Can you work these out from the drawing? Everything is in mm from the part's minimum corner. A direction names the side the tool comes from. Coordinates: 2 decimals unless noted, no trailing zeros. Write each loop counter-clockwise with the first axis right and the second up, starting at its lowest first coordinate (ties: lowest second). Pieces come first, ordered by that corner, then holes.
(1) Which directions (+Z, -Z, +X, -X, +Y, -Y) give clear straight access to the entire face, cutting with the end or side of a thin tool? Please do the marked faces 1, 2 and 3.
(2) Thinking about a two-plate mould opening in X: for the marked faces 4, 5, 6 and 7, which applies, released by +X, released by -X, zero draft, split by the parting line, or undercut?
(3) For pin 1 Ø3 at (y, z) = (1, 7.5) entering from +X; pin 2 Ø1.5 at (y, z) = (5, 2.5) entering from -X; pin 3 Ø1.5 at (x, y) = (2.5, 3) entering from -Z; pin 4 Ø1 at (y, z) = (1, 1.5) entering from -X, each with a flat end and sliding along its axis, tell me the tip position at first contact or that it passes through.
(4) Please list where these lines run through material, in increasing order: probe 1 along Z at (x, y) = (0.75, 3); probe 2 along Z at (x, y) = (4.25, 5.25); probe 3 along Y at (x, z) = (3.25, 5).
(5) Imagine slicing it at B-B, the plane x = 0.75. List the corners of the cut face in (y, z) for me.
(6) Imagine slicing it at A-A, the plane z = 5.5. List the corners of the cut face in (x, y) for me.
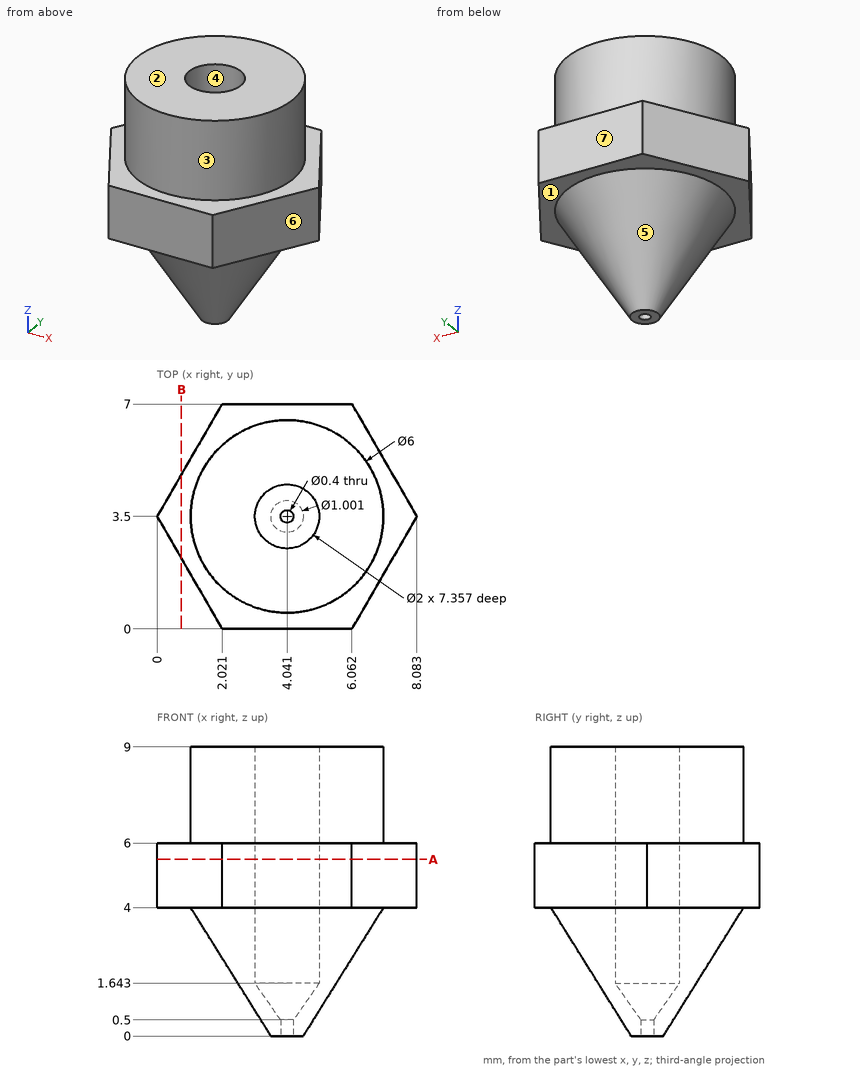
Recorded:
1. face 1: -Z
1. face 2: +Z, +X, -X, +Y, -Y
1. face 3: +Z
2. face 4: undercut
2. face 5: split by the parting line
2. face 6: released by +X
2. face 7: zero draft
3. pin 1: stops at x = 6.87
3. pin 2: stops at x = 1.84
3. pin 3: stops at z = 0.59
3. pin 4: passes through
4. probe 1: z = 4 to 6
4. probe 2: z = 2.02 to 9
4. probe 3: y = 0 to 2.89, 4.11 to 7
5. outline: (2.2, 4) - (4.8, 4) - (4.8, 6) - (2.2, 6) - close
6. outline: (0, 3.5) - (2.02, 0) - (6.06, 0) - (8.08, 3.5) - (6.06, 7) - (2.02, 7) - close; hole circle Ø2 at (4.04, 3.5)
